Verification items for the finished model (mm, model axes). A direction names the side the tool comes from. Round coordinates to 2 decimals unless told otherwise and drop trailing zeros. Write each loop counter-clockwise with the first axis right and the second up, starting at its lowest first coordinate (ties: lowest second). Pieces come first, ordered by that corner, then holes. Notation, with made-up numbers: (74.5, -15.5) - (87.5, -15.5) arc R17 ccw to (87.5, -2.5) - close; hole circle Ø6 at (79, -32). An arc over 180 degrees is marked (long way). Answer as a JSON object with one key per item and string values.
```python
from build123d import *

# Parameters (mm, degrees)
CYLINDER024_R          = 1.6
CYLINDER024_DEPTH      = 23
CYLINDER010_R          = 1.6
CYLINDER010_DEPTH      = 200
CYLINDER010_ROLL_ANGLE = 90
SKETCH006_W            = 50
SKETCH006_H            = 50
PAD009_DEPTH           = 3
SKETCH005_R            = 1.6
PAD008_DEPTH           = 7


with BuildPart() as cilindro024:
    # Cylinder024 → Cylinder024 (new body)
    with BuildSketch(Plane(origin=(220, 40, -41.5), x_dir=(1, 0, 0), z_dir=(0, 0, 1))):
        Circle(CYLINDER024_R)
    extrude(amount=CYLINDER024_DEPTH)


with BuildPart() as cilindro010:
    # Cylinder010 → Cylinder010 (new body)
    with BuildSketch(Plane.XY):
        Circle(CYLINDER010_R)
    extrude(amount=CYLINDER010_DEPTH)


with BuildPart() as cilindro010_1:
    # Cylinder010 roll: moved
    add(cilindro010.part.rotate(Axis((0, 0, 0), (1, 0, 0)), CYLINDER010_ROLL_ANGLE))


with BuildPart() as cilindro010_2:
    # Cylinder010 placement: moved
    add(cilindro010_1.part.moved(Location((220, 100, -34.5))))


with BuildPart() as pad009:
    # Sketch006 → Pad009 (new body, symmetric)
    with BuildSketch(Plane.XY):
        with Locations((203, 28)):
            Rectangle(SKETCH006_W, SKETCH006_H)
    extrude(amount=PAD009_DEPTH, both=True)


with BuildPart() as cut020:
    # Sketch005 → Pad008 (new body, symmetric)
    with BuildSketch(Plane.XY):
        with BuildLine():
            ThreePointArc((213.146217, 35.873783), (222.141241, 32.291882), (228, 40.000021))
            Line((228, 58.000021), (228, 40.000021))
            Line((228, 58.000021), (212, 58.000021))
            ThreePointArc((201.31003, 49.825331), (208.674868, 51.271332), (212, 58.000021))
            ThreePointArc((201.31003, 49.825331), (195.001272, 44.887217), (201.526329, 40.238664))
            ThreePointArc((213.146217, 35.873783), (208.095475, 40.07732), (201.526329, 40.238664))
        make_face()
        with Locations((200, 45)):
            Circle(SKETCH005_R, mode=Mode.SUBTRACT)
    extrude(amount=PAD008_DEPTH, both=True)

    # Cut005: cut Pad009
    add(pad009.part, mode=Mode.SUBTRACT)


with BuildPart() as cut020_1:
    # Cut005 placement: moved
    add(cut020.part.moved(Location((0, 0, -34.5))))

    # Cut006: cut Cilindro010
    add(cilindro010_2.part, mode=Mode.SUBTRACT)

    # Cut020: cut Cilindro024
    add(cilindro024.part, mode=Mode.SUBTRACT)


with BuildPart() as part_mirroring:
    # Part__Mirroring: instance of Cut020
    add(cut020_1.part.mirror(Plane(origin=(0, 0, 0), x_dir=(1, 0, 0), z_dir=(0, 1, 0))))


solid = part_mirroring.part
```
Q1. Section check C-C, the plane z = -34.5. Record the cut outline in (x, y).
Geometry check:
{"outline": "(210.37, -53) arc R8.47 cw to (212, -58) - (218.4, -58) - (218.4, -53) - close; (221.6, -58) - (228, -58) - (228, -53) - (221.6, -53) - close"}
Q2. Section check B-B, the plane y = -45. Record the cut outline in (x, z), then the cut area to 3 significant figures.
Geometry check:
{"outline": "(195, -41.5) - (198.4, -41.5) - (198.4, -37.5) - (195, -37.5) - close; (195, -31.5) - (198.4, -31.5) - (198.4, -27.5) - (195, -27.5) - close; (201.6, -41.5) - (228, -41.5) - (228, -37.5) - (201.6, -37.5) - close; (201.6, -31.5) - (228, -31.5) - (228, -27.5) - (201.6, -27.5) - close", "area": "238 mm2"}
Q3. Release check for a two-part mould opening along X. For faces 3 (the flat face through (228, -49, -38)), 4 (the flat face through (215, -45, -27.5)), 5 (the cylindrical face through (201.48, -44.39, -39.53)) record: released by +X, released by -X, zero draft, split by the parting line, or undercut.
Geometry check:
{"face 3": "released by +X", "face 4": "zero draft", "face 5": "undercut"}
Q4. Gauge pin test, flat ends, axial feed: P1, Ø4, axis at x = 220, y = -40, coming from the +Z side; P2, Ø2, axis at x = 216.5, z = -30.5, coming from the +Y side; P3, Ø6, axis at y = -35, z = -30, coming from the +X side; P4, Ø3, axis at x = 207, z = -31.5, coming from the +Y side. Record the tip position at first contact, or that the pin passes through.
Geometry check:
{"P1": "stops at z = -27.5", "P2": "stops at y = -32.4", "P3": "stops at x = 227.75", "P4": "stops at y = -39.92"}
Q5. Set-up check for faces 1 (the cylindrical face through (208.183, -40.044, -29.472)), 2 (the flat face through (215, -45, -31.5)): record each of +Z, -Z, +X, -X, +Y, -Y from which the full face is reachable in a straight line by a thin tool's end or side.
Geometry check:
{"face 1": "+Z, -Z, +Y", "face 2": "+X, -X, +Y"}
Q6. Section check D-D, the plane x = 200. Record the cut outline in (y, z), then the cut area to 3 significant figures.
Geometry check:
{"outline": "(-50, -41.5) - (-46.6, -41.5) - (-46.6, -37.5) - (-50, -37.5) - close; (-50, -31.5) - (-46.6, -31.5) - (-46.6, -27.5) - (-50, -27.5) - close; (-43.4, -41.5) - (-40, -41.5) - (-40, -37.5) - (-43.4, -37.5) - close; (-43.4, -31.5) - (-40, -31.5) - (-40, -27.5) - (-43.4, -27.5) - close", "area": "54.4 mm2"}
Q7. Material ranges on line 1 along Z through (x, y) = (220, -54.95); line 2 along Z through (x, y) = (207, -47.5); line 3 along Y through (x, z) = (220, -39.9), recorded low to high. Write a range as [from, to].
Geometry check:
{"line 1": "z = [-41.5, -36.1], [-32.9, -27.5]", "line 2": "z = [-41.5, -37.5], [-31.5, -27.5]", "line 3": "y = [-58, -41.6], [-38.4, -32]"}
Q8. Section check A-A, the plane x = 220. Record the cut outline in (y, z).
Geometry check:
{"outline": "(-58, -41.5) - (-41.6, -41.5) - (-41.6, -37.5) - (-53, -37.5) - (-53, -36.1) - (-58, -36.1) - close; (-58, -32.9) - (-53, -32.9) - (-53, -31.5) - (-41.6, -31.5) - (-41.6, -27.5) - (-58, -27.5) - close; (-38.4, -41.5) - (-32, -41.5) - (-32, -37.5) - (-38.4, -37.5) - close; (-38.4, -31.5) - (-32, -31.5) - (-32, -27.5) - (-38.4, -27.5) - close"}
